Can you work these out from the drawing? Everything is in mm from the part's minimum corner. A direction names the side the tool comes from. Round coordinates to 2 decimals unless told otherwise and drop trailing zeros. Write each loop counter-clockwise with the first axis right and the second up, starting at its lowest first coordinate (ties: lowest second). Pieces come first, ordered by that corner, then holes. Notation, with made-up numbers: (9.25, -16) -> (50.25, -16) arc R15 ccw to (50.25, -1) -> close; hole circle Ø6 at (74.5, 68.25). An arc over 180 degrees is marked (long way). Write item = value, one per line. Start each with the question number.
1) For the marked faces 1, 2, 3 and 4, which set-ups out of +Z, -Z, +X, -X, +Y, -Y let a thin tool reach every point of the face, with its end or its side?
2) I'm going to push flat-ended pins straight in: pin 1 (10 mm diameter, centred on y = 11.5, z = 8, fed in from -X); pin 2 (9.5 mm diameter, centred on x = 44, z = 32, fed in from -Y); pin 3 (4 mm diameter, centred on x = 61, z = 16, fed in from -Y). Where does each tip first touch, or does it pass through?
3) Imagine slicing it at C-C, the plane z = 8. State how many separate pieces and enclosed holes the cut face has, then the cut area to 3 significant figures.
4) Imagine slicing it at A-A, the plane y = 37.5. Please give me the cut outline in (x, z) (1 decimal).
5) If I drill on line 1 (Y direction, x = 41, z = 30); line 2 (Z direction, x = 27, y = 63); line 3 (Z direction, x = 54, y = 17), over which ranges is the centre line in solid material (lowest first)?
6) Thinking about a two-plate mould opening in Y: for the marked faces 5, 6, 7 and 8, which applies, +Y half, -Y half, draft (parallel to the pull), parting line (faces both ways), or undercut?
7) Imagine slicing it at D-D, the plane y = 4. Please give me the cut outline in (x, z), then the cut area to 3 significant figures.
8) Imagine slicing it at B-B, the plane x = 64. Please give me the cut outline in (y, z), then the cut area to 3 significant figures.
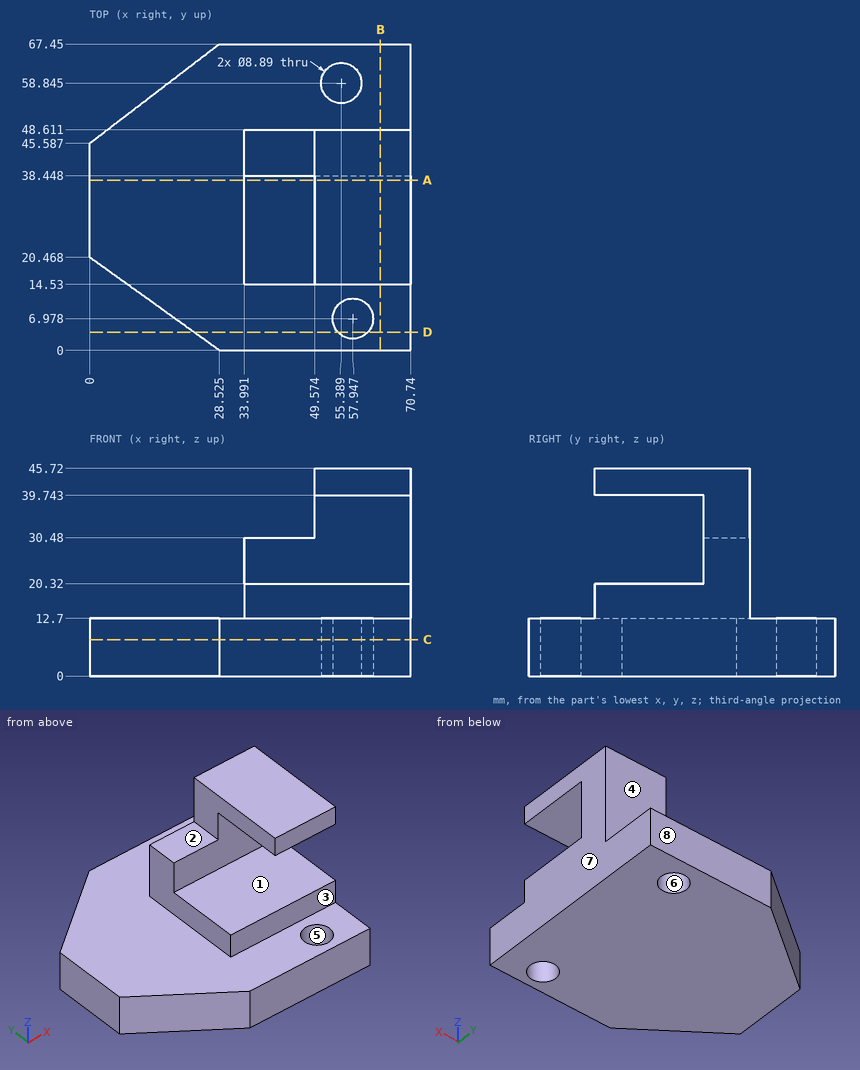
Reported:
q1.face_1 = +X, -X, -Y
q1.face_2 = +Z, -X, +Y, -Y
q1.face_3 = +Z, +X, -X, -Y
q1.face_4 = +Z, +X, -X, +Y
q2.pin_1 = 5.53
q2.pin_2 = 38.45
q2.pin_3 = 14.53
q3.separate_pieces = 1
q3.enclosed_holes = 2
q3.area = 4,040 mm²
q4.outline = (0, 0) -> (70.7, 0) -> (70.7, 20.3) -> (34, 20.3) -> (34, 12.7) -> (0, 12.7) -> close; (49.6, 39.7) -> (70.7, 39.7) -> (70.7, 45.7) -> (49.6, 45.7) -> close
q5.line_1 = 38.45 to 48.61
q5.line_2 = 0 to 12.7
q5.line_3 = 0 to 20.32, 39.74 to 45.72
q6.face_5 = undercut
q6.face_6 = undercut
q6.face_7 = draft
q6.face_8 = +Y half
q7.outline = (22.95, 0) -> (54.65, 0) -> (54.65, 12.7) -> (22.95, 12.7) -> close; (61.25, 0) -> (70.74, 0) -> (70.74, 12.7) -> (61.25, 12.7) -> close
q7.area = 523 mm²
q8.outline = (0, 0) -> (67.45, 0) -> (67.45, 12.7) -> (48.61, 12.7) -> (48.61, 45.72) -> (14.53, 45.72) -> (14.53, 39.74) -> (38.45, 39.74) -> (38.45, 20.32) -> (14.53, 20.32) -> (14.53, 12.7) -> (0, 12.7) -> close
q8.area = 1,520 mm²
